Autodesk Inventor part; units mm, degrees
ref_plane "Work Plane1" through (0, 10, 38.1) normal (0, 0, 1) x (1, 0, 0)
ref_plane "YZ Plane" through (0, 0, 0) normal (1, 0, 0) x (0, 1, 0)
ref_plane "XZ Plane" through (0, 0, 0) normal (0, 1, 0) x (-1, 0, 0)
sketch "Sketch1" plane through (0, 0, 0) normal (1, 0, 0) x (0, 1, 0)
  line L0 (0, 0) -> (50.8, 0) construction
  line L1 (50.8, 0) -> (50.8, 76.2) construction
  line L2 (50.8, 76.2) -> (0, 76.2) construction
  line L3 (0, 76.2) -> (0, 0) construction
  line L4 (40.8, 3.175) -> (10, 3.175)
  line L5 (10, 3.175) -> (10, 11.6)
  line L6 (10, 11.6) -> (3.175, 11.6)
  line L7 (3.175, 11.6) -> (3.175, 64.6)
  line L8 (3.175, 64.6) -> (10, 64.6)
  line L9 (10, 64.6) -> (10, 73.025)
  line L10 (10, 73.025) -> (40.8, 73.025)
  line L11 (40.8, 73.025) -> (40.8, 64.6)
  line L12 (40.8, 64.6) -> (47.625, 64.6)
  line L13 (47.625, 64.6) -> (47.625, 11.6)
  line L14 (47.625, 11.6) -> (40.8, 11.6)
  line L15 (40.8, 3.175) -> (40.8, 11.6)
  line L16 (25.4, 73.025) -> (25.4, 76.2) construction
  line L17 (47.625, 38.1) -> (50.8, 38.1) construction
  line L18 (3.175, 38.1) -> (0, 38.1) construction
  line L19 (25.4, 3.175) -> (25.4, 0) construction
  point P0 (1.5875, 38.1)
  dimension "d0" = 50.8
  dimension "d1" = 76.2
  dimension "d2" = 3.175
  dimension "d3" = 26.5
  dimension "d4" = 10
extrude "Extrusion1" add sketch "Sketch1" along normal blind 16
sketch "Sketch2" plane through (0, 10, 73.025) normal (0, 0, 1) x (1, 0, 0)
  line L0 (0, -10) -> (16, -10) construction
  line L1 (16, -10) -> (16, 40.8) construction
  line L2 (16, 40.8) -> (0, 40.8) construction
  line L3 (0, 40.8) -> (0, -10) construction
  circle A0 centre (8, 25.4) radius 3.175
  circle A1 centre (8, 5.4) radius 3.175
  line L4 (8, 25.4) -> (8, 40.8) construction
  line L5 (8, 5.4) -> (8, -10) construction
  dimension "d7" = 16
  dimension "d8" = 50.8
  dimension "d9" = 6.35
  dimension "d10" = 20
extrude "Extrusion2" cut sketch "Sketch2" against normal blind 16
ref_plane "Work Plane1" through (0, 10, 38.1) normal (0, 0, 1) x (1, 0, 0)
mirror "Mirror1" about plane through (0, 10, 38.1) normal (0, 0, 1) of "Extrusion2"
sketch "Sketch5" plane through (0, 47.625, 64.6) normal (0, 1, 0) x (1, 0, 0)
  line L0 (0, 64.6) -> (16, 64.6) construction
  line L1 (16, 64.6) -> (16, -11.6) construction
  line L2 (16, -11.6) -> (0, -11.6) construction
  line L3 (0, -11.6) -> (0, 64.6) construction
  line L4 (12.5, 3.4) -> (12.5, -11.6) construction
  line L5 (12.5, 49.6) -> (12.5, 64.6) construction
  line L6 (7.5, 8.4) -> (16, 8.4)
  line L7 (16, 8.4) -> (16, -11.6)
  line L8 (16, -11.6) -> (7.5, -11.6)
  line L9 (7.5, -11.6) -> (7.5, 8.4)
  line L10 (12.5, 3.4) -> (7.5, 3.4) construction
  line L11 (12.5, 3.4) -> (16, 3.4) construction
  line L12 (12.5, 3.4) -> (12.5, 8.4) construction
  line L13 (7.5, 44.6) -> (16, 44.6)
  line L14 (16, 44.6) -> (16, 64.6)
  line L15 (16, 64.6) -> (7.5, 64.6)
  line L16 (7.5, 64.6) -> (7.5, 44.6)
  line L17 (12.5, 49.6) -> (12.5, 44.6) construction
  line L18 (12.5, 49.6) -> (7.5, 49.6) construction
  dimension "d18" = 76.2
  dimension "d19" = 16
  dimension "d21" = 15
  dimension "d22" = 12.5
  dimension "d23" = 5
extrude "Extrusion4" cut sketch "Sketch5" against normal up to surface (6.825 mm away)
sketch "Sketch6" plane through (0, 3.175, 11.6) normal (0, -1, 0) x (1, 0, 0)
  line L0 (0, -11.6) -> (16, -11.6) construction
  line L1 (16, -11.6) -> (16, 64.6) construction
  line L2 (16, 64.6) -> (0, 64.6) construction
  line L3 (0, 64.6) -> (0, -11.6) construction
  line L4 (10, 53) -> (10, 0) construction
  line L5 (10, 26.5) -> (0, 26.5) construction
  line L6 (16, 43) -> (0, 43)
  line L7 (0, 43) -> (0, 64.6)
  line L8 (0, 64.6) -> (16, 64.6)
  line L9 (16, 64.6) -> (16, 43)
  line L10 (16, 10) -> (0, 10)
  line L11 (0, 10) -> (0, -11.6)
  line L12 (0, -11.6) -> (16, -11.6)
  line L13 (16, -11.6) -> (16, 10)
  dimension "d26" = 16
  dimension "d27" = 76.2
  dimension "d28" = 10
  dimension "d29" = 53
  dimension "d30" = 10
extrude "Extrusion5" cut sketch "Sketch6" against normal up to surface (6.825 mm away)
fillet "Fillet1" radius 3.5 6 edges at (8, 10, 54.6) (3.75, 40.8, 64.6) (11.75, 40.8, 56.2) (3.75, 40.8, 11.6) (11.75, 40.8, 20) (8, 10, 21.6)
sketch "Sketch4" plane through (0, 0, 0) normal (-1, 0, 0) x (0, 0, 1)
  line L0 (0, 0) -> (76.2, 0)
  line L1 (76.2, 0) -> (76.2, 50.8)
  line L2 (76.2, 50.8) -> (0, 50.8)
  line L3 (0, 50.8) -> (0, 0)
  dimension "d13" = 76.2
  dimension "d14" = 50.8
extrude "Extrusion3" add sketch "Sketch4" along normal blind 8
sketch "Sketch7" plane through (-8, 0, 0) normal (-1, 0, 0) x (0, 0, 1)
  circle A0 centre (38.1, 25.4) radius 14.5
  circle A1 centre (38.1, 25.4) radius 19 construction
  circle A2 centre (24.665, 38.835) radius 2.3
  circle A3 centre (38.1, 44.4) radius 2.3
  circle A4 centre (24.665, 11.965) radius 2.3
  circle A5 centre (38.1, 6.4) radius 2.3
  circle A6 centre (51.535, 38.835) radius 2.3
  circle A7 centre (51.535, 11.965) radius 2.3
  line L0 (51.535, 38.835) -> (38.1, 25.4) construction
  line L1 (38.1, 25.4) -> (38.1, 44.4) construction
  line L2 (0, 0) -> (76.2, 0) construction
  line L3 (76.2, 0) -> (76.2, 50.8) construction
  line L4 (76.2, 50.8) -> (0, 50.8) construction
  line L5 (0, 50.8) -> (0, 0) construction
  circle A8 centre (9.75, 25.4) radius 3.175
  circle A9 centre (66.45, 25.4) radius 3.175
  line L6 (9.75, 25.4) -> (0, 25.4) construction
  line L7 (66.45, 25.4) -> (76.2, 25.4) construction
  circle A10 centre (38.1, 25.4) radius 25 construction
  line L8 (18.1, 25.4) -> (9.75, 25.4) construction
  line L9 (38.1, 25.4) -> (18.1, 25.4) construction
  point P0 (38.1, 50.8)
  dimension "d37" = 29
  dimension "d38" = 38
  dimension "d39" = 4.6
  dimension "d40" = 45
  dimension "d41" = 76.2
  dimension "d42" = 50.8
  dimension "d43" = 6.35
  dimension "d44" = 6.35
  dimension "d45" = 50
  dimension "d51" = 20
  dimension "d52" = 8.35
extrude "Extrusion6" cut sketch "Sketch7" against normal through all
fillet "Fillet2" radius 3.175 4 edges at (-4, 50.8, 0) (-4, 50.8, 76.2) (-4, 0, 76.2) (-4, 0, 0)
properties part number "BS_Face" material "Aluminum 6061"
Can you work these out from the model? Positions are in its coordinate system, mm. A direction names the side the tool comes from. Coordinates: 2 decimals unless noted, no trailing zeros. Loops run counter-clockwise (first coordinate to the right, second up) from the corner with the lowest first, then second, coordinate; pieces in that order, holes last. Notation, with made-up numbers: (-18.5, 61.25) -> (-4.5, 61.25) arc R32 ccw to (-4.5, 94.25) -> close; hole circle Ø5 at (30, -2). An arc over 180 degrees is marked (long way). Put each result on its own line as item: value. Start each with the question number.
Q1. I want a section at D-D (x = 13.5). Count the separate pieces of the cut face and the enclosed holes in it, plus the area to 3 significant figures.
Q2. Thinking about a two-plate mould opening in X: for faces 5 (the face through (8, 35, 19.175)), 6 (the face through (16, 10, 39)), 7 (the face through (3.832, 40.774, 25.901)), which applies, pulls with the +X half, pulls with the -X half, needs draft (parallel to the pull), parting line crosses it, or undercut?
Q3. I want a section at B-B (y = 35.4). Write out the boundary of the cut face in (x, z) (3 decimals).
Q4. For faces 1 (the face through (10, 40.8, 8)), 2 (the face through (8, 47.625, 38)), 3 (the face through (8, 10, 11)), 4 (the face through (3.8, 41.8, 65.65)), which set-ups out of +Z, -Z, +X, -X, +Y, -Y let a thin tool reach every point of the face, with its end or its side?
Q5. If I drill on line 1 (Y direction, x = 8, z = 69.75) (3 decimals); line 2 (Z direction, x = 2.25, y = 26) (3 decimals); line 3 (X direction, y = 6, z = 14), over which ranges is the centre line in solid material (lowest first)? Write a range as [from, to].
Q6. I want a section at A-A (z = 38.1). Write out the boundary of the cut face in (x, y) (3 decimals).
Q7. I want a section at C-C (z = 9.75). Write out the boundary of the cut face in (x, y) (3 decimals), plus the area to 3 significant figures.
Q8. I'm going to push flat-ended pins straight in: P1, Ø3, axis at x = 8.5, y = 15.5, coming from the +Z side (3 decimals); P2, Ø1, axis at x = 13, y = 45.5, coming from the -Z side; P3, Ø6, axis at y = 11.965, z = 51.535, coming from the -X side; P4, Ø4, axis at x = 6, y = 6, coming from the +Z side. Where does each tip first touch, or does it pass through?
Taken from the geometry:
1. separate pieces: 1
1. enclosed holes: 9
1. area: 1,810 mm2
2. face 5: undercut
2. face 6: pulls with the +X half
2. face 7: needs draft
3. outline: (-8, 0) -> (0, 0) -> (0, 3.175) -> (4.825, 3.175) -> (4.825, 19.175) -> (11.175, 19.175) -> (11.175, 3.175) -> (16, 3.175) -> (16, 27.6) -> (-8, 27.6) -> close; (-8, 48.6) -> (16, 48.6) -> (16, 73.025) -> (11.175, 73.025) -> (11.175, 57.025) -> (4.825, 57.025) -> (4.825, 73.025) -> (0, 73.025) -> (0, 76.2) -> (-8, 76.2) -> close
4. face 1: -Z, +X, +Y
4. face 2: +Z, -Z, +X, +Y
4. face 3: -Z, +X, -Y
4. face 4: +Z, +X, +Y
5. line 1: y = [10, 12.225], [18.575, 32.225], [38.575, 40.8]
5. line 2: z = [3.175, 6.632], [12.868, 23.612], [52.588, 63.332], [69.568, 73.025]
5. line 3: x = [-8, 0]
6. outline: (-8, 0) -> (0, 0) -> (0, 3.175) -> (16, 3.175) -> (16, 4.1) -> (-8, 4.1) -> close; (-8, 8.7) -> (16, 8.7) -> (16, 10.9) -> (-8, 10.9) -> close; (-8, 39.9) -> (16, 39.9) -> (16, 42.1) -> (-8, 42.1) -> close; (-8, 46.7) -> (16, 46.7) -> (16, 47.625) -> (0, 47.625) -> (0, 50.8) -> (-8, 50.8) -> close
7. outline: (-8, 0) -> (0, 0) -> (0, 10) -> (16, 10) -> (16, 22.225) -> (-8, 22.225) -> close; (-8, 28.575) -> (16, 28.575) -> (16, 40.8) -> (7.5, 40.8) -> (7.5, 41.213) -> (0, 41.213) -> (0, 50.8) -> (-8, 50.8) -> close; hole circle Ø6.35 at (8, 15.4); hole circle Ø6.35 at (8, 35.4)
7. area: 687 mm2
8. P1: stops at z = 57.025
8. P2: stops at z = 20
8. P3: stops at x = -8
8. P4: stops at z = 54.94
